Geometry check sheet. Reference: the model listing, model coordinates, mm. Face numbers are marked on the shaded views. A direction names the side the tool comes from. Give positions to 0.01 mm unless a question says otherwise; leave off trailing zeros. Write each loop counter-clockwise with the first axis right and the second up, starting at its lowest first coordinate (ties: lowest second). Pieces come first, ordered by that corner, then holes. Notation, with made-up numbers: (38.5, 7) - (65.5, 7) arc R26 cw to (65.5, 44) - close; hole circle Ø7 at (61, 10.5). An arc over 180 degrees is marked (long way). Write item = value, one per line. Start each with the question number.
(1) Access from +Z, -Z, +X, -X, +Y, -Y to the whole of each face (thin tool, end or side, straight path). Record for the marked faces 1, 2 and 3.
(2) Section check D-D, the plane x = 0. Enter the section's corners in (y, z).
(3) Thickness scan on L1, parallel to Y at x = -13, z = 7.5; L2, parallel to Z at x = -4.5, y = 13; L3, parallel to Z at x = -2.5, y = -7.5. Record the ranges inside material, lowest first.
(4) Section check A-A, the plane x = -13. Enter the section's corners in (y, z), plus the area to 3 significant figures.
(5) Depth check by flat-ended pin: pin 1 Ø1.8 at (x, y) = (13, -13) entering from -Z; pin 2 Ø1.5 at (x, y) = (9, -7.5) entering from -Z; pin 3 Ø6 at (x, y) = (-13, 0) entering from +Z; pin 4 Ø17.5 at (x, y) = (-0.5, 3) entering from +Z. Enter the tip coordinate at first touch or a pass-through.
(6) Section check B-B, the plane z = 2. Enter the section's corners in (x, y), plus the area to 3 significant figures.
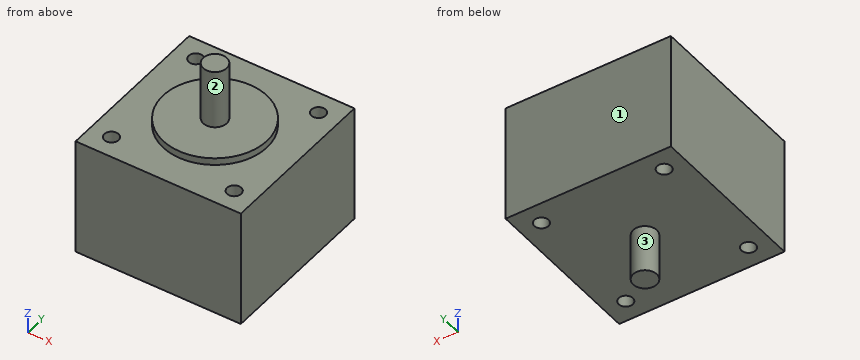
```python
from build123d import *

# Parameters (mm, degrees)
SKETCH1_W           = 35
SKETCH1_H           = 35
SKETCH1_R           = 1.5
BOSS_EXTRUDE1_DEPTH = 25
SKETCH2_R           = 11
BOSS_EXTRUDE2_DEPTH = 1.5
SKETCH3_R           = 2.5
BOSS_EXTRUDE3_DEPTH = 12.5
SKETCH4_R           = 2.5
BOSS_EXTRUDE4_DEPTH = 10


with BuildPart() as part:
    # Sketch1 → Boss-Extrude1 (new body)
    with BuildSketch(Plane.XY):
        Rectangle(SKETCH1_W, SKETCH1_H)
        with Locations((-13, 13)):
            Circle(SKETCH1_R, mode=Mode.SUBTRACT)
        with Locations((13, 13)):
            Circle(SKETCH1_R, mode=Mode.SUBTRACT)
        with Locations((-13, -13)):
            Circle(SKETCH1_R, mode=Mode.SUBTRACT)
        with Locations((13, -13)):
            Circle(SKETCH1_R, mode=Mode.SUBTRACT)
    extrude(amount=BOSS_EXTRUDE1_DEPTH)

    # Sketch2 → Boss-Extrude2 (add)
    with BuildSketch(Plane.XY.offset(25)):
        Circle(SKETCH2_R)
    extrude(amount=BOSS_EXTRUDE2_DEPTH)

    # Sketch3 → Boss-Extrude3 (add)
    with BuildSketch(Plane.XY.offset(26.5)):
        Circle(SKETCH3_R)
    extrude(amount=BOSS_EXTRUDE3_DEPTH)

    # Sketch4 → Boss-Extrude4 (add)
    with BuildSketch(Plane(origin=(0, 0, 0), x_dir=(-1, 0, 0), z_dir=(0, 0, -1))):
        Circle(SKETCH4_R)
    extrude(amount=BOSS_EXTRUDE4_DEPTH)


solid = part.part
```
Model answer:
q1.face_1 = +Z, -Z, +X, -X, +Y
q1.face_2 = +Z
q1.face_3 = -Z
q2.outline = (-17.5, 0) - (-2.5, 0) - (-2.5, -10) - (2.5, -10) - (2.5, 0) - (17.5, 0) - (17.5, 25) - (11, 25) - (11, 26.5) - (2.5, 26.5) - (2.5, 39) - (-2.5, 39) - (-2.5, 26.5) - (-11, 26.5) - (-11, 25) - (-17.5, 25) - close
q3.L1 = -17.5 to -14.5, -11.5 to 11.5, 14.5 to 17.5
q3.L2 = 0 to 25
q3.L3 = 0 to 26.5
q4.outline = (-17.5, 0) - (-14.5, 0) - (-14.5, 25) - (-17.5, 25) - close; (-11.5, 0) - (11.5, 0) - (11.5, 25) - (-11.5, 25) - close; (14.5, 0) - (17.5, 0) - (17.5, 25) - (14.5, 25) - close
q4.area = 725 mm²
q5.pin_1 = through
q5.pin_2 = 0
q5.pin_3 = 26.5
q5.pin_4 = 39
q6.outline = (-17.5, -17.5) - (17.5, -17.5) - (17.5, 17.5) - (-17.5, 17.5) - close; hole circle Ø3 at (-13, -13); hole circle Ø3 at (-13, 13); hole circle Ø3 at (13, -13); hole circle Ø3 at (13, 13)
q6.area = 1,200 mm²
